Input: part model. Units: mm. Frame: model coordinates. Coordinates: 2 decimals unless noted, no trailing zeros. Write each loop counter-clockwise with the first axis right and the second up, starting at its lowest first coordinate (ties: lowest second). Pieces come first, ordered by that corner, then holes. Notation, with made-up numbers: M -13,7 L 4,7 A25 ccw 4,28 Z; hole C 26,23.25 d4. An arc over 180 degrees is marked long. Use one line per item in the form item = value.
from build123d import *

# Parameters (mm, degrees)
BOSS_EXTRUDE1_DEPTH               = 6.35
CUT_EXTRUDE1_REACH                = 463.209
SKETCH3_R                         = 14.2875
SKETCH3_R_2                       = 19.05
SKETCH3_R_3                       = 2.413
SKETCH3_R_4                       = 3.96875
F_3_8_CLEARANCE_HOLE2_D           = 9.8044
F_3_8_CLEARANCE_HOLE2_CSINK_D     = 11.58748
F_3_8_CLEARANCE_HOLE2_CSINK_ANGLE = 90
F_1_4_0_2500_DOWEL_HOLE2_D        = 6.35


with BuildPart() as part:
    # Sketch2 → Boss-Extrude1 (new body)
    with BuildSketch(Plane(origin=(0, 0, 0), x_dir=(0, 0, -1), z_dir=(1, 0, 0))):
        with BuildLine():
            Line((-420.65776111, -67.281464584), (-373.03276111, 59.718535416))
            ThreePointArc((-373.03276111, 59.718535416), (-370.505449055, 64.705606261), (-366.948304567, 69.018946606))
            Line((-366.948304567, 69.018946606), (-255.966736674, 176.828999095))
            ThreePointArc((-255.966736674, 176.828999095), (-237.853043868, 185.216470627), (-218.467902472, 180.454975186))
            Line((-218.467902472, 180.454975186), (17.349576345, 26.590500195))
            ThreePointArc((17.349576345, 26.590500195), (27.457947121, -15.941255906), (-14.489671706, -28.250874568))
            ThreePointArc((-14.489671706, -28.250874568), (-207.31672278, 0.568286884), (-378.160809237, -93.373790032))
            ThreePointArc((-378.160809237, -93.373790032), (-410.165032474, -97.845670164), (-420.65776111, -67.281464584))
        make_face()
    extrude(amount=BOSS_EXTRUDE1_DEPTH)

    # Sketch3 → Cut-Extrude1 (cut, up to next)
    with BuildSketch(Plane(origin=(6.35, 0, 0), x_dir=(0, 0, -1), z_dir=(1, 0, 0)), mode=Mode.PRIVATE) as cut_extrude1_sk1:
        with Locations((-203.2, 111.125)):
            Circle(SKETCH3_R)
    cut_extrude1_tool1 = extrude(cut_extrude1_sk1.sketch, amount=-CUT_EXTRUDE1_REACH, mode=Mode.PRIVATE) & part.part
    # Sketch3 → Cut-Extrude1 (cut, up to next)
    with BuildSketch(Plane(origin=(6.35, 0, 0), x_dir=(0, 0, -1), z_dir=(1, 0, 0)), mode=Mode.PRIVATE) as cut_extrude1_sk2:
        with Locations((-349.25, 50.8)):
            Circle(SKETCH3_R)
    cut_extrude1_tool2 = extrude(cut_extrude1_sk2.sketch, amount=-CUT_EXTRUDE1_REACH, mode=Mode.PRIVATE) & part.part
    # Sketch3 → Cut-Extrude1 (cut, up to next)
    with BuildSketch(Plane(origin=(6.35, 0, 0), x_dir=(0, 0, -1), z_dir=(1, 0, 0)), mode=Mode.PRIVATE) as cut_extrude1_sk3:
        with Locations((-396.875, -76.2)):
            Circle(SKETCH3_R)
    cut_extrude1_tool3 = extrude(cut_extrude1_sk3.sketch, amount=-CUT_EXTRUDE1_REACH, mode=Mode.PRIVATE) & part.part
    # Sketch3 → Cut-Extrude1 (cut, up to next)
    with BuildSketch(Plane(origin=(6.35, 0, 0), x_dir=(0, 0, -1), z_dir=(1, 0, 0)), mode=Mode.PRIVATE) as cut_extrude1_sk4:
        with Locations((-234.95, 155.194)):
            Circle(SKETCH3_R_2)
    cut_extrude1_tool4 = extrude(cut_extrude1_sk4.sketch, amount=-CUT_EXTRUDE1_REACH, mode=Mode.PRIVATE) & part.part
    # Sketch3 → Cut-Extrude1 (cut, up to next)
    with BuildSketch(Plane(origin=(6.35, 0, 0), x_dir=(0, 0, -1), z_dir=(1, 0, 0)), mode=Mode.PRIVATE) as cut_extrude1_sk5:
        with Locations((-252.910512242, 137.233487758)):
            Circle(SKETCH3_R_3)
    cut_extrude1_tool5 = extrude(cut_extrude1_sk5.sketch, amount=-CUT_EXTRUDE1_REACH, mode=Mode.PRIVATE) & part.part
    # Sketch3 → Cut-Extrude1 (cut, up to next)
    with BuildSketch(Plane(origin=(6.35, 0, 0), x_dir=(0, 0, -1), z_dir=(1, 0, 0)), mode=Mode.PRIVATE) as cut_extrude1_sk6:
        with Locations((-216.989487758, 137.233487758)):
            Circle(SKETCH3_R_4)
    cut_extrude1_tool6 = extrude(cut_extrude1_sk6.sketch, amount=-CUT_EXTRUDE1_REACH, mode=Mode.PRIVATE) & part.part
    # Sketch3 → Cut-Extrude1 (cut, up to next)
    with BuildSketch(Plane(origin=(6.35, 0, 0), x_dir=(0, 0, -1), z_dir=(1, 0, 0)), mode=Mode.PRIVATE) as cut_extrude1_sk7:
        with Locations((-216.989487758, 173.154512242)):
            Circle(SKETCH3_R_3)
    cut_extrude1_tool7 = extrude(cut_extrude1_sk7.sketch, amount=-CUT_EXTRUDE1_REACH, mode=Mode.PRIVATE) & part.part
    # Sketch3 → Cut-Extrude1 (cut, up to next)
    with BuildSketch(Plane(origin=(6.35, 0, 0), x_dir=(0, 0, -1), z_dir=(1, 0, 0)), mode=Mode.PRIVATE) as cut_extrude1_sk8:
        with Locations((-252.910512242, 173.154512242)):
            Circle(SKETCH3_R_4)
    cut_extrude1_tool8 = extrude(cut_extrude1_sk8.sketch, amount=-CUT_EXTRUDE1_REACH, mode=Mode.PRIVATE) & part.part
    add(cut_extrude1_tool1.solids().sort_by_distance((6.35, 111.125, 203.2))[0], mode=Mode.SUBTRACT)
    add(cut_extrude1_tool2.solids().sort_by_distance((6.35, 50.8, 349.25))[0], mode=Mode.SUBTRACT)
    add(cut_extrude1_tool3.solids().sort_by_distance((6.35, -76.2, 396.875))[0], mode=Mode.SUBTRACT)
    add(cut_extrude1_tool4.solids().sort_by_distance((6.35, 155.194, 234.95))[0], mode=Mode.SUBTRACT)
    add(cut_extrude1_tool5.solids().sort_by_distance((6.35, 137.233488, 252.910512))[0], mode=Mode.SUBTRACT)
    add(cut_extrude1_tool6.solids().sort_by_distance((6.35, 137.233488, 216.989488))[0], mode=Mode.SUBTRACT)
    add(cut_extrude1_tool7.solids().sort_by_distance((6.35, 173.154512, 216.989488))[0], mode=Mode.SUBTRACT)
    add(cut_extrude1_tool8.solids().sort_by_distance((6.35, 173.154512, 252.910512))[0], mode=Mode.SUBTRACT)

    # 3/8 Clearance Hole2 (through all)
    with Locations(Plane(origin=(6.35, 0, 0), x_dir=(0, 0, -1), z_dir=(1, 0, 0))):
        with Locations((0, 0)):
            CounterSinkHole(F_3_8_CLEARANCE_HOLE2_D / 2, F_3_8_CLEARANCE_HOLE2_CSINK_D / 2, counter_sink_angle=F_3_8_CLEARANCE_HOLE2_CSINK_ANGLE)

    # 1/4 (0.2500) Dowel Hole2 (through all)
    with Locations(Plane(origin=(6.35, 0, 0), x_dir=(0, 0, -1), z_dir=(1, 0, 0))):
        with Locations((-271.4625, -6.35)):
            Hole(F_1_4_0_2500_DOWEL_HOLE2_D / 2)


solid = part.part
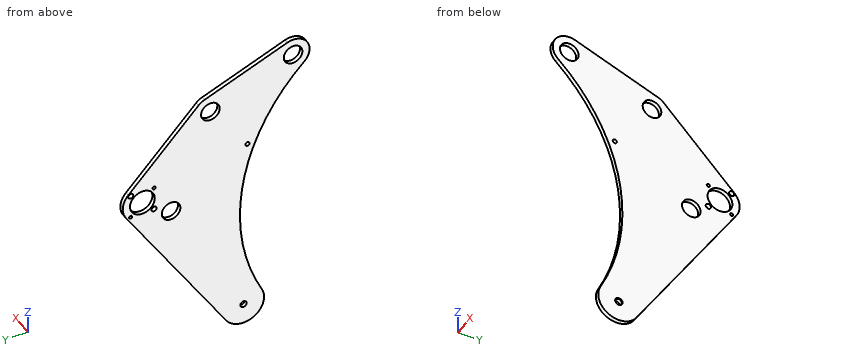
(1) Section query B-B on y = -23. Return the cut outline in (x, z).
Computed:
outline = M 0,-21.89 L 6.35,-21.89 L 6.35,25.24 L 0,25.24 Z; M 0,281.94 L 6.35,281.94 L 6.35,404.05 L 0,404.05 Z
(2) Section query A-A on z = 0. Return the cut outline in (x, y).
Computed:
outline = M 0,-31.75 L 6.35,-31.75 L 6.35,-5.79 L 5.46,-4.9 L 0,-4.9 Z; M 0,4.9 L 5.46,4.9 L 6.35,5.79 L 6.35,37.91 L 0,37.91 Z
(3) Section query D-D on z = 349.25. Return the cut outline in (x, y).
Computed:
outline = M 0,-65.75 L 6.35,-65.75 L 6.35,36.51 L 0,36.51 Z; M 0,65.09 L 6.35,65.09 L 6.35,86.21 L 0,86.21 Z
(4) Section query C-C on x = 2. State how many separate pieces and enclosed holes the cut face has, plus the area to 3 significant figures.
Computed:
separate_pieces = 1
enclosed_holes = 10
area = 53,900 mm^2
(5) Line query: probe 1 along Y at (x, z) = (2, 349.25); probe 2 along Z at (x, y) = (4.5, 149.5); probe 3 along Y at (x, z) = (2, 0). Output: solid intervals per line, ascending.
Computed:
probe_1 = -65.75 to 36.51, 65.09 to 86.21
probe_2 = 171.03 to 216.77, 253.13 to 284.1
probe_3 = -31.75 to -4.9, 4.9 to 37.91
(6) First-contact query: pin 1 Ø1 at (x, y) = (1, 5.5) entering from +Z. Flat tip, straight axial feed; report the tip coordinate or a pass-through.
Computed:
pin_1 = 393.55
